Geometry: see drawing. Coordinates: mm, zero at the bounding-box minimum. A direction names the side the tool comes from. Coordinates: 2 decimals unless noted, no trailing zeros. Loops run counter-clockwise (first coordinate to the right, second up) from the corner with the lowest first, then second, coordinate; pieces in that order, holes last.
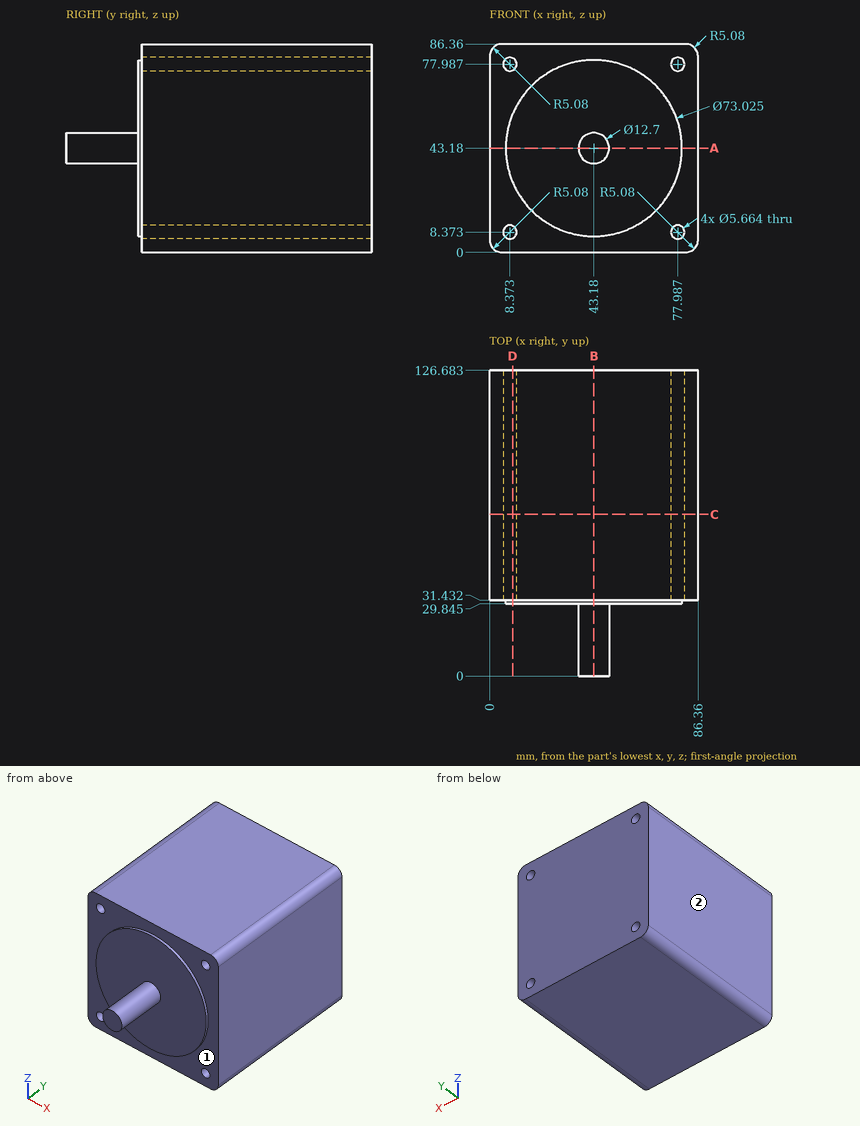
Item 1: Contact query for flat-ended pins moving along their axis: P1, Ø6.5, axis at x = 8.37, z = 77.99, coming from the -Y side; P2, Ø22, axis at x = 57.5, z = 59.5, coming from the -Y side (1 decimal); P3, Ø6.5, axis at x = 77.99, z = 8.37, coming from the +Y side. Output: stop coordinate, or through.
Result:
P1: stops at y = 31.43
P2: stops at y = 29.8
P3: stops at y = 126.68
Item 2: Section query B-B (x = 43.18). Output: boundary loops of the cut face in (y, z) (1 decimal), then the cut area to 3 significant figures.
Result:
outline: (0, 36.8) - (29.8, 36.8) - (29.8, 6.7) - (31.4, 6.7) - (31.4, 0) - (126.7, 0) - (126.7, 86.4) - (31.4, 86.4) - (31.4, 79.7) - (29.8, 79.7) - (29.8, 49.5) - (0, 49.5) - close
area: 8,720 mm2
Item 3: Section query A-A (z = 43.18). Output: boundary loops of the cut face in (x, y) (1 decimal).
Result:
outline: (0, 31.4) - (6.7, 31.4) - (6.7, 29.8) - (36.8, 29.8) - (36.8, 0) - (49.5, 0) - (49.5, 29.8) - (79.7, 29.8) - (79.7, 31.4) - (86.4, 31.4) - (86.4, 126.7) - (0, 126.7) - close
Item 4: Section query C-C (y = 67). Output: boundary loops of the cut face in (x, z) (1 decimal).
Result:
outline: (0, 5.1) arc R5.1 ccw to (5.1, 0) - (81.3, 0) arc R5.1 ccw to (86.4, 5.1) - (86.4, 81.3) arc R5.1 ccw to (81.3, 86.4) - (5.1, 86.4) arc R5.1 ccw to (0, 81.3) - close; hole circle Ø5.7 at (8.4, 8.4); hole circle Ø5.7 at (8.4, 78); hole circle Ø5.7 at (78, 8.4); hole circle Ø5.7 at (78, 78)
Item 5: Reachability of the marked faces 1 and 2 from +Z, -Z, +X, -X, +Y, -Y: full face, straight path, thin tool, end or side. Return the list, or none.
Result:
face 1: -Y
face 2: +Z, -Z, -X, +Y, -Y
Item 6: Line query: L1, parallel to X at y = 51, z = 76.5; L2, parallel to Y at x = 50, z = 50.5 (1 decimal); L3, parallel to X at y = 48.5, z = 81.5 (1 decimal). Output: solid intervals per line, ascending.
Result:
L1: x = 0 to 5.96, 10.78 to 75.58, 80.4 to 86.36
L2: y = 29.8 to 126.7
L3: x = 0 to 86.4
Item 7: Section query D-D (x = 9.5). Output: boundary loops of the cut face in (y, z) (1 decimal), then the cut area to 3 significant figures.
Result:
outline: (29.8, 29.1) - (31.4, 29.1) - (31.4, 11) - (126.7, 11) - (126.7, 75.4) - (31.4, 75.4) - (31.4, 57.3) - (29.8, 57.3) - close; (31.4, 0) - (126.7, 0) - (126.7, 5.8) - (31.4, 5.8) - close; (31.4, 80.6) - (126.7, 80.6) - (126.7, 86.4) - (31.4, 86.4) - close
area: 7,280 mm2
